Part model, mm, in its own coordinate system. A direction names the side the tool comes from. Coordinates: 2 decimals unless noted, no trailing zeros. Loops run counter-clockwise (first coordinate to the right, second up) from the corner with the lowest first, then second, coordinate; pieces in that order, holes last. Notation, with made-up numbers: (51.25, 13) -> (100.25, 13) arc R26 cw to (100.25, 39) -> close; hole circle Ø8 at (22.5, 45). An arc over 180 degrees is marked (long way). Use one line per item in the form item = value. Start each with the question number.
(1) Band-saw the part on C-C on y = 10.5. Give the cut face in (x, z), then the cut area to 3 significant figures.
(2) 3-axis set-ups, long thin cutter, end or side, ignore diameter. For faces 1 (the flat face through (-0.3, -30.65, 19.7)), 2 (the flat face through (0, 0, 37)): which of +Z, -Z, +X, -X, +Y, -Y reach the whole face in a straight line?
(3) Drill centre lines: L1, parallel to Y at x = -8, z = 29.5; L2, parallel to X at y = -28, z = 14; L3, parallel to Z at x = -14.5, y = 4. Where is each one in solid material? Low to high. Write a range as [from, to].
(4) Band-saw the part on A-A on x = 8.5. Give the cut face in (y, z), then the cut area to 3 significant figures.
(5) Pin check, flat tips, straight feed: P1, Ø3, axis at y = -15, z = 34.5, coming from the -X side; P2, Ø6, axis at y = -12, z = 34.5, coming from the +X side; P3, Ø7.5, axis at x = -9, y = 9, coming from the -Z side. Stop position of each tip, or through.
(6) Band-saw the part on B-B on z = 14.47. Give the cut face in (x, y) (3 decimals), then the cut area to 3 significant figures.
(7) Band-saw the part on D-D on x = -1. Give the cut face in (y, z), then the cut area to 3 significant figures.
(8) Mould opens along Z. For faces 3 (the flat face through (10, 28, 20)), 4 (the flat face through (-15, 0, 38)), 5 (the flat face through (-7, 0, 35)), 6 (the cylindrical face through (13.756, -28.185, 14.6)) say: +Z half, -Z half, draft (parallel to the pull), parting line (faces both ways), or undercut.
```python
from build123d import *

# Parameters (mm, degrees)
SKETCH_1_W          = 40
SKETCH_1_H          = 61.3
EXTRUDE_1_DEPTH     = 40
SKETCH_2_W          = 20
SKETCH_2_H          = 51.3
CUT_EXTRUDE_1_DEPTH = 55.216441233
SKETCH_3_W          = 5
SKETCH_3_H          = 51.3
CUT_EXTRUDE_2_DEPTH = 55.216441233
SKETCH_4_W          = 35
SKETCH_4_H          = 51.3
CUT_EXTRUDE_3_DEPTH = 55.216441233
SKETCH_5_W          = 20
SKETCH_5_H          = 20
CUT_EXTRUDE_5_DEPTH = 76.879443857
SKETCH_6_R          = 1
CUT_EXTRUDE_6_DEPTH = 76.879443857


with BuildPart() as part:
    # 草图1 → 凸台-拉伸1 (new body)
    with BuildSketch(Plane.XY):
        Rectangle(SKETCH_1_W, SKETCH_1_H)
    extrude(amount=EXTRUDE_1_DEPTH)

    # 草图2 → 切除-拉伸1 (cut, through all)
    with BuildSketch(Plane.XY.offset(40)):
        with Locations((10, 0)):
            Rectangle(SKETCH_2_W, SKETCH_2_H)
    extrude(amount=-CUT_EXTRUDE_1_DEPTH, mode=Mode.SUBTRACT)

    # 草图3 → 切除-拉伸2 (cut, through all)
    with BuildSketch(Plane.XY.offset(40)):
        with Locations((-17.5, 0)):
            Rectangle(SKETCH_3_W, SKETCH_3_H)
    extrude(amount=-CUT_EXTRUDE_2_DEPTH, mode=Mode.SUBTRACT)

    # 草图4 → 切除-拉伸3 (cut, through all)
    with BuildSketch(Plane(origin=(0, 0, 0), x_dir=(0, 0, -1), z_dir=(1, 0, 0))):
        with Locations((-17.5, 0)):
            Rectangle(SKETCH_4_W, SKETCH_4_H)
    extrude(amount=-CUT_EXTRUDE_3_DEPTH, mode=Mode.SUBTRACT)

    # 草图5 → 切除-拉伸5 (cut, through all)
    with BuildSketch(Plane.XZ.offset(30.65)):
        with BuildLine():
            ThreePointArc((-19.697451431, 36.307856046), (-19.923182678, 36.885031943), (-20, 37.5))
            Line((-20, 37.5), (-20, 36.865536816))
            Line((-20, 36.865536816), (-19.697451431, 36.307856046))
        make_face()
        with BuildLine():
            ThreePointArc((-20, 37.5), (-19.267766953, 39.267766953), (-17.5, 40))
            Line((-17.5, 40), (-20, 40))
            Line((-20, 40), (-20, 37.5))
        make_face()
        Polygon((0, 0), (-19.697451431, 36.307856046), (-20, 36.865536816), (-20, 0), align=None)
        with Locations((10, 30)):
            Rectangle(SKETCH_5_W, SKETCH_5_H)
    extrude(amount=-CUT_EXTRUDE_5_DEPTH, mode=Mode.SUBTRACT)

    # 草图6 → 切除-拉伸6 (cut, through all)
    with BuildSketch(Plane.XZ.offset(30.65)):
        with Locations(Location((12.765, 14.47, 0), (0, 0, 270))):
            Circle(SKETCH_6_R)
        with Locations(Location((17.237135955, 5.52572809, 0), (0, 0, 270))):
            Circle(SKETCH_6_R)
    extrude(amount=-CUT_EXTRUDE_6_DEPTH, mode=Mode.SUBTRACT)


solid = part.part
```
A:
q1.outline = (-15, 35) -> (0, 35) -> (0, 40) -> (-15, 40) -> close
q1.area = 75.0 mm²
q2.face_1 = +Z, -Z, +X, -X, -Y
q2.face_2 = +Z, +X, +Y, -Y
q3.L1 = [-30.65, -25.65], [25.65, 30.65]
q3.L2 = [-7.6, 11.88], [13.65, 20]
q3.L3 = [35, 40]
q4.outline = (-30.65, 0) -> (-25.65, 0) -> (-25.65, 20) -> (-30.65, 20) -> close; (25.65, 0) -> (30.65, 0) -> (30.65, 20) -> (25.65, 20) -> close
q4.area = 200 mm²
q5.P1 = -15
q5.P2 = 0
q5.P3 = 35
q6.outline = (-7.85, -30.65) -> (11.765, -30.65) -> (11.765, -25.65) -> (-7.85, -25.65) -> close; (-7.85, 25.65) -> (11.765, 25.65) -> (11.765, 30.65) -> (-7.85, 30.65) -> close; (13.765, -30.65) -> (20, -30.65) -> (20, -25.65) -> (13.765, -25.65) -> close; (13.765, 25.65) -> (20, 25.65) -> (20, 30.65) -> (13.765, 30.65) -> close
q6.area = 259 mm²
q7.outline = (-30.65, 1.84) -> (-25.65, 1.84) -> (-25.65, 35) -> (25.65, 35) -> (25.65, 1.84) -> (30.65, 1.84) -> (30.65, 40) -> (-30.65, 40) -> close
q7.area = 638 mm²
q8.face_3 = +Z half
q8.face_4 = draft
q8.face_5 = -Z half
q8.face_6 = undercut
